Here's how the part is built. I have some questions about the finished solid (model axes, mm). Face numbers are marked on the shaded views. A direction names the side the tool comes from. Coordinates: 2 decimals unless noted, no trailing zeros. Write each loop counter-clockwise with the first axis right and the second up, starting at its lowest first coordinate (ties: lowest second). Pieces come first, ordered by that corner, then holes.
```python
from build123d import *

# Parameters (mm, degrees)
F0_R     = 31.75
F1_DEPTH = 44.45
F2_R     = 12.7
F3_DEPTH = 12.7
F4_R     = 5.08


with BuildPart() as f1:
    # F0 (on Top) → F1 (new body)
    with BuildSketch(Plane.XY):
        with Locations((-9.30992, 5.807177)):
            Circle(F0_R)
    extrude(amount=F1_DEPTH)

    # F2 (on face) → F3 (join)
    with BuildSketch(Plane.XY.offset(44.45)):
        with Locations((-9.30992, 5.807177)):
            Circle(F2_R)
    extrude(amount=F3_DEPTH)

    # F4
    f4_edges = [f1.edges().sort_by_distance(p)[0] for p in [
        (-41.05992, 5.807177, 44.45),
        (-41.05992, 5.807177, 0),
        (-22.00992, 5.807177, 57.15),
    ]]
    fillet(f4_edges, radius=F4_R)


solid = f1.part
```
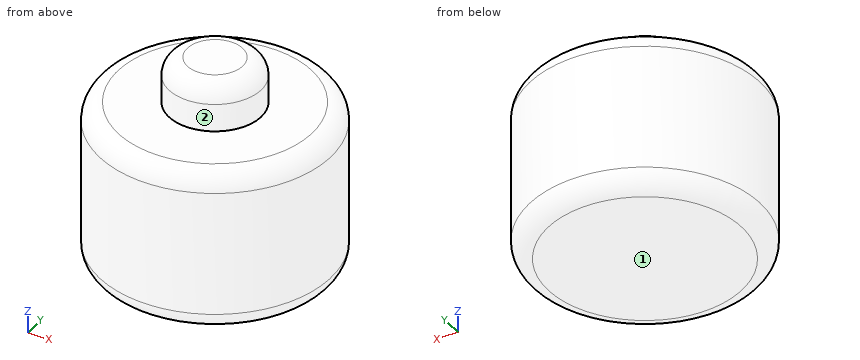
1) On a 3-axis mill with a long thin cutter (end or side, diameter ignored), from which of +Z, -Z, +X, -X, +Y, -Y can I reach the whole of each face in a straight line? I mean the marked faces 1 and 2. Say none if no direction works.
Values follow:
face 1: -Z, +X, -X, +Y, -Y
face 2: +Z
2) Imagine slicing it at B-B on z = 18.5. Please give me the cut outline in (x, y), then the cut area to 3 significant figures.
Values follow:
outline: circle Ø63.5 at (-9.31, 5.81)
area: 3,170 mm2
3) I need wall thicknesses on probe 1 along Z at (x, y) = (-30, 2); probe 2 along X at (y, z) = (-16, 32.5); probe 3 along Y at (x, z) = (-31.5, 25.5). Which ranges of each line are inside material? Lowest first, please.
Values follow:
probe 1: z = 0 to 44.45
probe 2: x = -32.39 to 13.77
probe 3: y = -16.9 to 28.52
4) Will these pins go through, and if not, where does the flat tip stop? pin 1 (1 mm diameter, centred on x = -32, y = 24.5, fed in from -Z); pin 2 (2 mm diameter, centred on x = 11, y = -16.5, fed in from +Z); pin 3 (5 mm diameter, centred on x = -15, z = 21, fed in from +Y).
Values follow:
pin 1: stops at z = 0.51
pin 2: stops at z = 43.79
pin 3: stops at y = 37.4
5) Imagine slicing it at A-A on z = 50. Please give me the cut outline in (x, y).
Values follow:
outline: circle Ø25.4 at (-9.31, 5.81)
